For this review, take the finished solid that the model builds, in its own axes (mm). Face numbers are marked on the shaded views. A direction names the side the tool comes from. Round coordinates to 2 decimals unless told otherwise and drop trailing zeros. Write each loop counter-clockwise with the first axis right and the second up, starting at its lowest first coordinate (ties: lowest second). Pieces come first, ordered by that corner, then holes. Notation, with made-up numbers: (-21, 52.5) - (-1, 52.5) arc R23 cw to (-1, 72.5) - close; hole circle Ø2 at (-22, -13.5). An arc over 180 degrees is marked (long way). One line per item, written item: value. Start each with the question number.
Q1. Add section D-D on x = 17.5. Write out the cut boundary in (y, z), and give its area (3 significant figures).
Q2. Clearance check with a flat-ended pin moving along its axis: pin 1 Ø3 at (x, y) = (25, 0) entering from -Z. State where the tip first meets the part, or that it passes through.
Q3. Add section B-B on z = 1.8. Write out the cut boundary in (x, y).
Q4. For probe 1 along X at (y, z) = (4, 2.3); probe 2 along Y at (x, z) = (-17.5, 3.05); probe 3 along X at (y, z) = (-1, 4.7), list the stretches that pass through material, from the lowest coordinate up.
Q5. Add section A-A on x = -25. Write out the cut boundary in (y, z), and give its area (3 significant figures).
Q6. Add section C-C on y = 0. Write out the cut boundary in (x, z).
Q7. Mouldability with a two-part tool opening along Y and no side actions: class the marked faces 3, 4 and 5 as +Y half, -Y half, draft (parallel to the pull), parting line (faces both ways), or undercut.
Q8. Tool access review of the marked faces 1 and 2: name each direction out of +Z, -Z, +X, -X, +Y, -Y from which nothing blocks a thin tool from reaching the whole face with its end or side.
```python
from build123d import *

# Parameters (mm, degrees)
SKETCH_W   = 57.4
SKETCH_H   = 19
SKETCH_R   = 1.7
SKETCH_W_2 = 42.6
SKETCH_H_2 = 11
PAD_DEPTH  = 5


with BuildPart() as part:
    # Sketch → Pad (new body)
    with BuildSketch(Plane.XY):
        Rectangle(SKETCH_W, SKETCH_H)
        with Locations((-25, 0)):
            Circle(SKETCH_R, mode=Mode.SUBTRACT)
        with Locations((25, 0)):
            Circle(SKETCH_R, mode=Mode.SUBTRACT)
        Rectangle(SKETCH_W_2, SKETCH_H_2, mode=Mode.SUBTRACT)
    extrude(amount=PAD_DEPTH)


solid = part.part
```
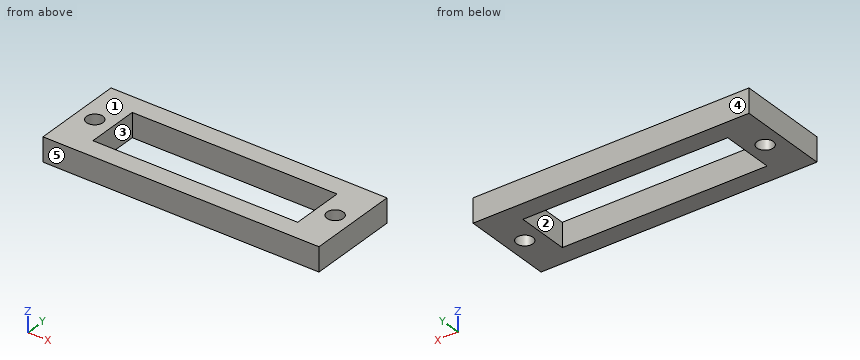
Result set:
1. outline: (-9.5, 0) - (-5.5, 0) - (-5.5, 5) - (-9.5, 5) - close; (5.5, 0) - (9.5, 0) - (9.5, 5) - (5.5, 5) - close
1. area: 40.0 mm^2
2. pin 1: passes through
3. outline: (-28.7, -9.5) - (28.7, -9.5) - (28.7, 9.5) - (-28.7, 9.5) - close; hole circle Ø3.4 at (-25, 0); hole (-21.3, -5.5) - (21.3, -5.5) - (21.3, 5.5) - (-21.3, 5.5) - close; hole circle Ø3.4 at (25, 0)
4. probe 1: x = -28.7 to -21.3, 21.3 to 28.7
4. probe 2: y = -9.5 to -5.5, 5.5 to 9.5
4. probe 3: x = -28.7 to -26.37, -23.63 to -21.3, 21.3 to 23.63, 26.37 to 28.7
5. outline: (-9.5, 0) - (-1.7, 0) - (-1.7, 5) - (-9.5, 5) - close; (1.7, 0) - (9.5, 0) - (9.5, 5) - (1.7, 5) - close
5. area: 78.0 mm^2
6. outline: (-28.7, 0) - (-26.7, 0) - (-26.7, 5) - (-28.7, 5) - close; (-23.3, 0) - (-21.3, 0) - (-21.3, 5) - (-23.3, 5) - close; (21.3, 0) - (23.3, 0) - (23.3, 5) - (21.3, 5) - close; (26.7, 0) - (28.7, 0) - (28.7, 5) - (26.7, 5) - close
7. face 3: undercut
7. face 4: +Y half
7. face 5: -Y half
8. face 1: +Z, +X, -X, +Y, -Y
8. face 2: +Z, -Z
